Read the model definition and answer for the solid it produces. Units are mm, in the model's axes. Give positions to 0.01 mm unless a question says otherwise; leave off trailing zeros. Write each loop counter-clockwise with the first axis right and the second up, starting at its lowest first coordinate (ties: lowest second). Pieces come first, ordered by that corner, then holes. Notation, with made-up numbers: (43.25, 60) - (76.25, 60) arc R16 cw to (76.25, 88) - close; hole circle Ø11 at (-33.5, 43). An arc over 180 degrees is marked (long way). Use CSV: the item, a comma, the result in double quotes. Start each with the question number.
from build123d import *

# Parameters (mm, degrees)
SKETCH1_W                  = 451
SKETCH1_H                  = 156.7072167
SKETCH1_W_2                = 431.95
SKETCH1_H_2                = 137.6572167
EXTRUDE_THIN1_DEPTH        = 4.7625
FILLET1_R                  = 2
F_10_CLEARANCE_HOLE1_D     = 4.9784
F_10_CLEARANCE_HOLE1_DEPTH = 9.525
F_10_24_TAPPED_HOLE1_D     = 3.7973
F_10_24_TAPPED_HOLE1_DEPTH = 250.46
F_10_24_TAPPED_HOLE1_TIP   = 1.140824014
F_10_CLEARANCE_HOLE2_D     = 5.1054
F_10_CLEARANCE_HOLE2_DEPTH = 20
F_10_CLEARANCE_HOLE2_TIP   = 1.533816902
F_10_24_TAPPED_HOLE2_D     = 3.7973
F_10_24_TAPPED_HOLE2_DEPTH = 14.95
F_10_24_TAPPED_HOLE2_TIP   = 1.140824014
F_10_24_TAPPED_HOLE3_D     = 3.7973
F_10_24_TAPPED_HOLE3_DEPTH = 14.95
F_10_24_TAPPED_HOLE3_TIP   = 1.140824014


with BuildPart() as part:
    # Sketch1 → Extrude-Thin1 (new body, symmetric)
    with BuildSketch(Plane(origin=(0, 0, 0), x_dir=(0, 0, -1), z_dir=(1, 0, 0))):
        Rectangle(SKETCH1_W, SKETCH1_H)
        Rectangle(SKETCH1_W_2, SKETCH1_H_2, mode=Mode.SUBTRACT)
    extrude(amount=EXTRUDE_THIN1_DEPTH, both=True)

    # Fillet1
    fillet1_edges = [part.edges().sort_by_distance(p)[0] for p in [
        (0, 68.82860835, 215.975),
        (0, -68.82860835, 215.975),
        (0, -68.82860835, -215.975),
        (0, 68.82860835, -215.975),
    ]]
    fillet(fillet1_edges, radius=FILLET1_R)

    # #10 Clearance Hole1
    with Locations(Plane(origin=(0, -68.82860835, 0), x_dir=(1, 0, 0), z_dir=(0, 1, 0))):
        with Locations((0, 206.45), (0, 0), (0, -206.45)):
            Hole(F_10_CLEARANCE_HOLE1_D / 2, depth=F_10_CLEARANCE_HOLE1_DEPTH)

    # #10-24 Tapped Hole1
    with Locations(Plane(origin=(0, 0, -225.5), x_dir=(-1, 0, 0), z_dir=(0, 0, -1))):
        with Locations((0, 40.25360835), (0, -40.25360835)):
            Hole(F_10_24_TAPPED_HOLE1_D / 2, depth=F_10_24_TAPPED_HOLE1_DEPTH)
            with Locations((0, 0, -(F_10_24_TAPPED_HOLE1_DEPTH + F_10_24_TAPPED_HOLE1_TIP / 2))):  # 118° drill point
                Cone(0, F_10_24_TAPPED_HOLE1_D / 2, F_10_24_TAPPED_HOLE1_TIP, mode=Mode.SUBTRACT)

    # #10 Clearance Hole2
    with Locations(Plane.XY.offset(225.5)):
        with Locations((0, 40.25360835), (0, -40.25360835)):
            Hole(F_10_CLEARANCE_HOLE2_D / 2, depth=F_10_CLEARANCE_HOLE2_DEPTH)
            with Locations((0, 0, -(F_10_CLEARANCE_HOLE2_DEPTH + F_10_CLEARANCE_HOLE2_TIP / 2))):  # 118° drill point
                Cone(0, F_10_CLEARANCE_HOLE2_D / 2, F_10_CLEARANCE_HOLE2_TIP, mode=Mode.SUBTRACT)

    # #10-24 Tapped Hole2
    with Locations(Plane.ZY.offset(4.7625)):
        with Locations((-190, 73.59110835), (-35, 73.59110835), (-190, -73.59110835), (35, -73.59110835), (190, -73.59110835), (190, 73.59110835)):
            Hole(F_10_24_TAPPED_HOLE2_D / 2, depth=F_10_24_TAPPED_HOLE2_DEPTH)
            with Locations((0, 0, -(F_10_24_TAPPED_HOLE2_DEPTH + F_10_24_TAPPED_HOLE2_TIP / 2))):  # 118° drill point
                Cone(0, F_10_24_TAPPED_HOLE2_D / 2, F_10_24_TAPPED_HOLE2_TIP, mode=Mode.SUBTRACT)

    # #10-24 Tapped Hole3
    with Locations(Plane(origin=(0, 78.35360835, 0), x_dir=(1, 0, 0), z_dir=(0, 1, 0))):
        with Locations((0, 206.45), (0, 0), (0, -206.45)):
            Hole(F_10_24_TAPPED_HOLE3_D / 2, depth=F_10_24_TAPPED_HOLE3_DEPTH)
            with Locations((0, 0, -(F_10_24_TAPPED_HOLE3_DEPTH + F_10_24_TAPPED_HOLE3_TIP / 2))):  # 118° drill point
                Cone(0, F_10_24_TAPPED_HOLE3_D / 2, F_10_24_TAPPED_HOLE3_TIP, mode=Mode.SUBTRACT)


solid = part.part
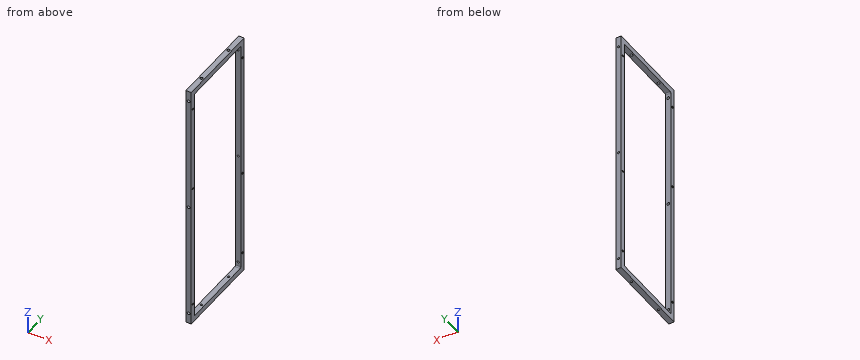
(1) The part is cut by section A-A on z = 132. Write down the section's boundary in (x, y).
(2) Given P1, Ø3.5, axis at y = 73.59, z = -190, coming from the -X side (3 decimals); P2, Ø4.5, axis at x = 0, z = 0, coming from the -Y side, each flat-ended and moving along its own axis, determine where each tip first touches the part or whether it passes through.
(3) Consider probe 1 along Y at (x, z) = (1.5, -35); probe 2 along Y at (x, z) = (1.25, -190); probe 3 along Y at (x, z) = (-1, 15). Determine where each line is inside the solid, lowest interval first.
(4) The part is cut by section B-B on y = 30.5. Write down the section's boundary in (x, z) (1 decimal), plus the area to 3 significant figures.
Reported:
1,outline,"(-4.76, -78.35) - (4.76, -78.35) - (4.76, -68.83) - (-4.76, -68.83) - close; (-4.76, 68.83) - (4.76, 68.83) - (4.76, 78.35) - (-4.76, 78.35) - close"
2,P1,"through"
2,P2,"y = 68.83"
3,probe 1,"-78.35 to -68.83, 68.83 to 71.69, 75.49 to 78.35"
3,probe 2,"-78.35 to -75.49, -71.69 to -68.83, 68.83 to 71.69, 75.49 to 78.35"
3,probe 3,"-78.35 to -68.83, 68.83 to 78.35"
4,outline,"(-4.8, -225.5) - (4.8, -225.5) - (4.8, -216) - (-4.8, -216) - close; (-4.8, 216) - (4.8, 216) - (4.8, 225.5) - (-4.8, 225.5) - close"
4,area,"181 mm²"
